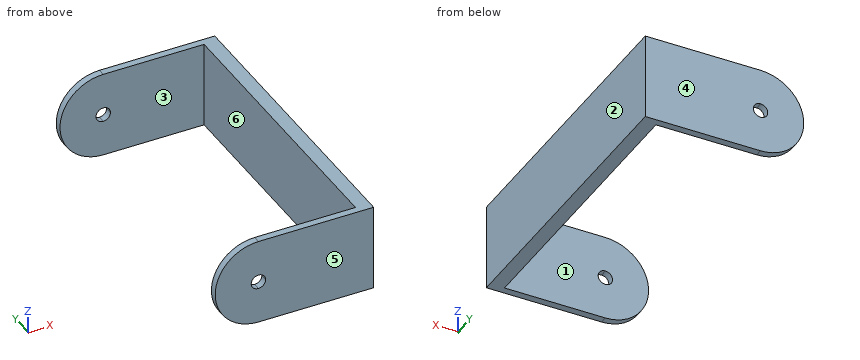
```python
from build123d import *

# Parameters (mm, degrees)
F1_DEPTH = 5.25
F2_W     = 3.5
F2_H     = 10
F2_W_2   = 2.3031880188
F3_DEPTH = 5


with BuildPart() as f1:
    # F0 (on Front) → F1 (new body, symmetric)
    with BuildSketch(Plane.XZ):
        with BuildLine():
            Line((3.2857142857, 1.5), (-0.7142857143, 1.5))
            ThreePointArc((-0.7142857143, 1.5), (0.3463744575, 1.0606601718), (0.7857142857, 0))
            ThreePointArc((0.7857142857, 0), (0.3463744575, -1.0606601718), (-0.7142857143, -1.5))
            Line((-0.7142857143, -1.5), (3.2857142857, -1.5))
            Line((3.2857142857, -1.5), (3.2857142857, 1.5))
        make_face()
        with BuildLine():
            ThreePointArc((0.7857142857, 0), (0.3463744575, 1.0606601718), (-0.7142857143, 1.5))
            Line((-0.7142857143, 1.5), (-0.7142857143, 0.25))
            ThreePointArc((-0.7142857143, 0.25), (-0.537509019, 0.1767766953), (-0.4642857143, 0))
            ThreePointArc((-0.4642857143, 0), (-0.537509019, -0.1767766953), (-0.7142857143, -0.25))
            Line((-0.7142857143, -0.25), (-0.7142857143, -1.5))
            ThreePointArc((-0.7142857143, -1.5), (0.3463744575, -1.0606601718), (0.7857142857, 0))
        make_face()
        with BuildLine():
            Line((-0.7142857143, 0.25), (-0.7142857143, 1.5))
            ThreePointArc((-0.7142857143, 1.5), (-2.2142857143, 0), (-0.7142857143, -1.5))
            Line((-0.7142857143, -1.5), (-0.7142857143, -0.25))
            ThreePointArc((-0.7142857143, -0.25), (-0.9642857143, 0), (-0.7142857143, 0.25))
        make_face()
    extrude(amount=F1_DEPTH, both=True)

    # F2 (on face) → F3 (cut, symmetric)
    with BuildSketch(Plane.XY.offset(1.5)):
        with Locations((1.0357142857, 0)):
            Rectangle(F2_W, F2_H)
        with Locations((-1.8658797237, 0)):
            Rectangle(F2_W_2, F2_H)
    extrude(amount=F3_DEPTH, both=True, mode=Mode.SUBTRACT)


solid = f1.part
```
The listing builds one solid part. Answer for the finished solid, in the listing's coordinates (mm). Face numbers are marked on the shaded views. A direction names the side the tool comes from. Give positions to 0.01 mm unless a question says otherwise; leave off trailing zeros. Order: outer loops, then holes, each group sorted by start corner. A loop starts at its lowest first (then second) coordinate and runs counter-clockwise, first axis right, second up. Notation, with made-up numbers: (25, 77.25) - (84, 77.25) arc R22 cw to (84, 92.25) - close; hole circle Ø11 at (1, 84). An arc over 180 degrees is marked (long way). Answer in a Markdown table with one row per item. Add a question column.
Q1. For a pull along Y with two mould halves and no side action, classify the marked faces 1, 2, 3 and 4 as released by +Y, released by -Y, zero draft, split by the parting line, or undercut.
Q2. Given P1, Ø0.9, axis at y = 2.5, z = 0.5, coming from the -X side, flat-ended and moving along its own axis, determine where the tip first touches the part or whether it passes through.
Q3. The part is cut by section B-B (z = -0.5). Determine the outline of the cut face in (x, y), then the cut area to 3 significant figures.
Q4. The part is cut by section C-C (y = 1.5). Determine the outline of the cut face in (x, z).
Q5. The part is cut by section D-D (z = 0.7). Determine the outline of the cut face in (x, y), then the cut area to 3 significant figures.
Q6. The part is cut by section A-A (x = 1.65). Determine the outline of the cut face in (y, z).
Q7. Find the intervals of material crossed by line 1 along Y through (x, z) = (0.05, -1.4); line 2 along X through (y, z) = (-0.5, -0.05), in increasing order. Write a range as [from, to].
Q8. Which of the six approach directions +Z, -Z, +X, -X, +Y, -Y give full straight-line access (tool end or side, diameter ignored) to the marked faces 5 and 6?
Determined:
| question | item | result |
|---|---|---|
| 1 | face 1 | undercut |
| 1 | face 2 | zero draft |
| 1 | face 3 | undercut |
| 1 | face 4 | released by +Y |
| 2 | P1 | stops at x = 2.79 |
| 3 | outline | (-2.13, -5.25) - (3.29, -5.25) - (3.29, 5.25) - (-2.13, 5.25) - (-2.13, 5) - (2.79, 5) - (2.79, -5) - (-2.13, -5) - close |
| 3 | area | 7.71 mm² |
| 4 | outline | (2.79, -1.5) - (3.29, -1.5) - (3.29, 1.5) - (2.79, 1.5) - close |
| 5 | outline | (-2.04, -5.25) - (3.29, -5.25) - (3.29, 5.25) - (-2.04, 5.25) - (-2.04, 5) - (2.79, 5) - (2.79, -5) - (-2.04, -5) - close |
| 5 | area | 7.66 mm² |
| 6 | outline | (-5.25, -1.5) - (-5, -1.5) - (-5, 1.5) - (-5.25, 1.5) - close; (5, -1.5) - (5.25, -1.5) - (5.25, 1.5) - (5, 1.5) - close |
| 7 | line 1 | y = [-5.25, -5], [5, 5.25] |
| 7 | line 2 | x = [2.79, 3.29] |
| 8 | face 5 | +Z, -Z, +X, -X, -Y |
| 8 | face 6 | +Z, -Z, -X |
